from build123d import *

# Parameters (mm, degrees)
SKETCH_1_W      = 40
SKETCH_1_H      = 9
SKETCH_1_R      = 2.1
EXTRUDE_1_DEPTH = 3
FILLET_1_R      = 2


with BuildPart() as part:
    # 草图1 → 凸台-拉伸1 (new body)
    with BuildSketch(Plane.XY):
        Rectangle(SKETCH_1_W, SKETCH_1_H)
        Circle(SKETCH_1_R, mode=Mode.SUBTRACT)
    extrude(amount=EXTRUDE_1_DEPTH)

    # 圆角1
    fillet_1_edges = [part.edges().sort_by_distance(p)[0] for p in [
        (-20, 4.5, 1.5),
        (20, 4.5, 1.5),
        (20, -4.5, 1.5),
        (-20, -4.5, 1.5),
    ]]
    fillet(fillet_1_edges, radius=FILLET_1_R)


solid = part.part
CAD build for the part. Positions are in the model's coordinates, mm. Round coordinates to 2 decimals unless told otherwise and drop trailing zeros. Loops run counter-clockwise (first coordinate to the right, second up) from the corner with the lowest first, then second, coordinate; pieces in that order, holes last.
(1) Wall check: line 1 along Y through (x, z) = (0, 2.35); line 2 along X through (y, z) = (1.75, 0.75); line 3 along Y through (x, z) = (-1, 1.7). Give the ranges that are in metal, low to high.
(2) Cut at B-B (z = 2.5). Give the cut face in (x, y).
(3) Cut at A-A (x = 0). Give the cut face in (y, z), plus the area to 3 significant figures.
(4) Cut at C-C (y = 0). Give the cut face in (x, z).
(5) Cut at D-D (y = 3.75). Give the cut face in (x, z).
Findings below:
1. line 1: y = -4.5 to -2.1, 2.1 to 4.5
1. line 2: x = -20 to -1.16, 1.16 to 20
1. line 3: y = -4.5 to -1.85, 1.85 to 4.5
2. outline: (-20, -2.5) arc R2 ccw to (-18, -4.5) - (18, -4.5) arc R2 ccw to (20, -2.5) - (20, 2.5) arc R2 ccw to (18, 4.5) - (-18, 4.5) arc R2 ccw to (-20, 2.5) - close; hole circle Ø4.2 at (0, 0)
3. outline: (-4.5, 0) - (-2.1, 0) - (-2.1, 3) - (-4.5, 3) - close; (2.1, 0) - (4.5, 0) - (4.5, 3) - (2.1, 3) - close
3. area: 14.4 mm2
4. outline: (-20, 0) - (-2.1, 0) - (-2.1, 3) - (-20, 3) - close; (2.1, 0) - (20, 0) - (20, 3) - (2.1, 3) - close
5. outline: (-19.56, 0) - (19.56, 0) - (19.56, 3) - (-19.56, 3) - close
